Verification items for this drawing (mm, ordinates from the low corner). A direction names the side the tool comes from. Coordinates: 2 decimals unless noted, no trailing zeros. Write each loop counter-clockwise with the first axis right and the second up, starting at its lowest first coordinate (ties: lowest second). Pieces come first, ordered by that corner, then holes. Notation, with made-up numbers: (77, -6.5) -> (87, -6.5) arc R26 cw to (87, 8.5) -> close; hole circle Ø9 at (68.25, -36.5). An arc over 180 degrees is marked (long way). Put each result on its own line as item: value. Start each with the question number.
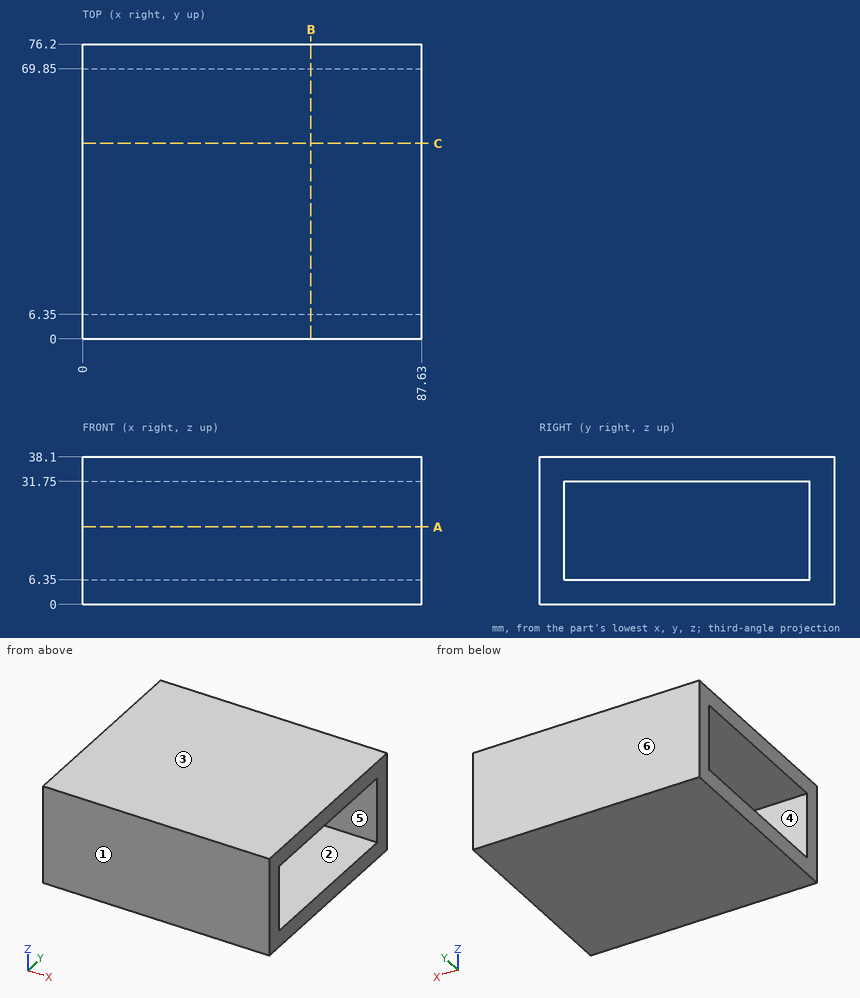
Item 1: Access from +Z, -Z, +X, -X, +Y, -Y to the whole of each face (thin tool, end or side, straight path). Record for the marked faces 1 and 2.
Item 2: Mould release check, pull along Y, two halves, no side actions. Record for the marked faces 3, 4, 5 and 6: released by +Y, released by -Y, zero draft, split by the parting line, or undercut.
Item 3: Section check B-B, the plane x = 59. Enter the section's corners in (y, z).
Item 4: Section check A-A, the plane z = 20. Enter the section's corners in (x, y).
Item 5: Section check C-C, the plane y = 50.5. Enter the section's corners in (x, z).
Item 6: Scan lines: line 1 along Z through (x, y) = (43, 66); line 2 along Y through (x, z) = (57.5, 28). Record each from-to range of solid material in increasing order. Write a range as [from, to].
Item 7: Go/stop test with a flat-tipped pin: P1, Ø10, axis at y = 9.5, z = 23.5, coming from the +X side. Record where the tip stops, or that it passes through.
From the geometry:
1. face 1: +Z, -Z, +X, -X, -Y
1. face 2: +X, -X
2. face 3: zero draft
2. face 4: undercut
2. face 5: undercut
2. face 6: released by +Y
3. outline: (0, 0) -> (76.2, 0) -> (76.2, 38.1) -> (0, 38.1) -> close; hole (6.35, 6.35) -> (69.85, 6.35) -> (69.85, 31.75) -> (6.35, 31.75) -> close
4. outline: (0, 0) -> (87.63, 0) -> (87.63, 6.35) -> (0, 6.35) -> close; (0, 69.85) -> (87.63, 69.85) -> (87.63, 76.2) -> (0, 76.2) -> close
5. outline: (0, 0) -> (87.63, 0) -> (87.63, 6.35) -> (0, 6.35) -> close; (0, 31.75) -> (87.63, 31.75) -> (87.63, 38.1) -> (0, 38.1) -> close
6. line 1: [0, 6.35], [31.75, 38.1]
6. line 2: [0, 6.35], [69.85, 76.2]
7. P1: x = 87.63
